from build123d import *

# Parameters (mm, degrees)
BOSS_EXTRUDE1_DEPTH = 1.475
BOSS_EXTRUDE2_DEPTH = 20


with BuildPart() as part:
    # Sketch1 → Boss-Extrude1 (new, symmetric)
    with BuildSketch(Plane.XY):
        Polygon((-29.75, 10), (-23, 10), (-23, -1.3), (-23, -2.8), (23, -2.8), (23, -1.3), (23, 10), (29.75, 10), (29.75, -10), (-29.75, -10), align=None)
    extrude(amount=BOSS_EXTRUDE1_DEPTH, both=True)

    # Sketch2 → Boss-Extrude2 (add)
    with BuildSketch(Plane.XY.offset(1.475)):
        Polygon((-23, -2.8), (23, -2.8), (24.5, -2.8), (24.5, -10), (23, -10), (-23, -10), (-24.5, -10), (-24.5, -2.8), align=None)
    extrude(amount=BOSS_EXTRUDE2_DEPTH)


solid = part.part
Verification items for the finished model (mm, model axes). A direction names the side the tool comes from. Coordinates: 2 decimals unless noted, no trailing zeros. Order: outer loops, then holes, each group sorted by start corner. A loop starts at its lowest first (then second) coordinate and runs counter-clockwise, first axis right, second up. Notation, with made-up numbers: M -29.5,43 L 29.5,43 A32 cw 29.5,79 Z; hole C 56,47.25 d11. An arc over 180 degrees is marked long. Write each question's results on one line, items separated by ' | '.
1) Section check A-A on y = 4.5. Record the cut outline in (x, z) (3 decimals).
Solved:
outline: M -29.75,-1.475 L -23,-1.475 L -23,1.475 L -29.75,1.475 Z; M 23,-1.475 L 29.75,-1.475 L 29.75,1.475 L 23,1.475 Z
2) Access from +Z, -Z, +X, -X, +Y, -Y to the whole of each face (thin tool, end or side, straight path). Record for faces 1 (the face through (23, 4, 0)), 2 (the face through (26, 10, 0)), 3 (the face through (24.5, -6, 11)).
Solved:
face 1: +Z, -Z, +Y | face 2: +Z, -Z, +X, -X, +Y | face 3: +Z, +X, +Y, -Y
3) Release check for a two-part mould opening along X. For faces 4 (the face through (-24.5, -6, 11)), 5 (the face through (-23, 4, 0)), 6 (the face through (0, -4, -1.475)) record: pulls with the +X half, pulls with the -X half, needs draft (parallel to the pull), parting line crosses it, or undercut.
Solved:
face 4: pulls with the -X half | face 5: undercut | face 6: needs draft
4) Scan lines: line 1 along X through (y, z) = (5.5, 0.5); line 2 along Y through (x, z) = (-17.5, 6.25); line 3 along X through (y, z) = (-7.75, 6.25). Record each from-to range of solid material in increasing order. Write a range as [from, to].
Solved:
line 1: x = [-29.75, -23], [23, 29.75] | line 2: y = [-10, -2.8] | line 3: x = [-24.5, 24.5]
5) Gauge pin test, flat ends, axial feed: pin 1 Ø1 at (x, z) = (18, 14) entering from +Y; pin 2 Ø8 at (y, z) = (-7, 15) entering from -X; pin 3 Ø6 at (y, z) = (-5, 7) entering from +X. Record the tip position at first contact, or that the pin passes through.
Solved:
pin 1: stops at y = -2.8 | pin 2: stops at x = -24.5 | pin 3: stops at x = 24.5
6) Section check C-C on z = 14. Record the cut outline in (x, y), plus the area to 3 significant figures.
Solved:
outline: M -24.5,-10 L 24.5,-10 L 24.5,-2.8 L -24.5,-2.8 Z | area: 353 mm²
7) Section check B-B on y = -7. Record the cut outline in (x, z) (3 decimals).
Solved:
outline: M -29.75,-1.475 L 29.75,-1.475 L 29.75,1.475 L 24.5,1.475 L 24.5,21.475 L -24.5,21.475 L -24.5,1.475 L -29.75,1.475 Z
8) Section check D-D on x = 14. Record the cut outline in (y, z) (3 decimals), plus the area to 3 significant figures.
Solved:
outline: M -10,-1.475 L -2.8,-1.475 L -2.8,21.475 L -10,21.475 Z | area: 165 mm²
